from build123d import *

# Parameters (mm, degrees)
SKETCH1_W              = 38.1
SKETCH1_H              = 25.4
BOSS_EXTRUDE1_DEPTH    = 22.225
F_10_CLEARANCE_HOLE1_D = 5.1054
CHAMFER1_SIZE          = 3.175
SKETCH6_W              = 6.35
SKETCH6_H              = 6.35
BOSS_EXTRUDE3_DEPTH    = 6.35
CUT_EXTRUDE1_REACH     = 38.753
SKETCH7_W              = 4.5
SKETCH7_H              = 3.175
CHAMFER4_SIZE          = 1.5875
CHAMFER5_SIZE          = 1.5875
FILLET2_R              = 0.79375


with BuildPart() as part:
    # Sketch1 → Boss-Extrude1 (new body)
    with BuildSketch(Plane(origin=(0, 0, 0), x_dir=(1, 0, 0), z_dir=(0, 1, 0))):
        Rectangle(SKETCH1_W, SKETCH1_H)
    extrude(amount=BOSS_EXTRUDE1_DEPTH)

    # #10 Clearance Hole1 (through all)
    with Locations(Plane(origin=(0, 22.225, 0), x_dir=(1, 0, 0), z_dir=(0, 1, 0))):
        with Locations((-12.7, 0), (12.7, 0)):
            Hole(F_10_CLEARANCE_HOLE1_D / 2)

    # Chamfer1
    chamfer1_edges = [part.edges().sort_by_distance(p)[0] for p in [
        (19.05, 11.1125, 12.7),
        (-19.05, 11.1125, 12.7),
        (-19.05, 11.1125, -12.7),
        (19.05, 11.1125, -12.7),
    ]]
    chamfer(chamfer1_edges, length=CHAMFER1_SIZE)

    # Sketch6 → Boss-Extrude3 (add)
    with BuildSketch(Plane.XY.offset(12.7)):
        with Locations((0, 3.175)):
            Rectangle(SKETCH6_W, SKETCH6_H)
    extrude(amount=BOSS_EXTRUDE3_DEPTH)

    # Sketch7 → Cut-Extrude1 (cut, up to next)
    with BuildSketch(Plane.ZY.offset(3.175), mode=Mode.PRIVATE) as cut_extrude1_sk1:
        with Locations((14.95, 3.175)):
            Rectangle(SKETCH7_W, SKETCH7_H)
    cut_extrude1_tool1 = extrude(cut_extrude1_sk1.sketch, amount=-CUT_EXTRUDE1_REACH, mode=Mode.PRIVATE) & part.part
    add(cut_extrude1_tool1.solids().sort_by_distance((-3.175, 3.175, 14.95))[0], mode=Mode.SUBTRACT)

    # Chamfer4
    chamfer4_edges = [part.edges().sort_by_distance(p)[0] for p in [
        (0, 0, 19.05),
        (0, 6.35, 19.05),
    ]]
    chamfer(chamfer4_edges, length=CHAMFER4_SIZE)

    # Chamfer5
    chamfer5_edges = [part.edges().sort_by_distance(p)[0] for p in [
        (-3.175, 5.55625, 12.7),
        (3.175, 0.79375, 12.7),
        (0, 6.35, 12.7),
        (3.175, 5.55625, 12.7),
        (-3.175, 0.79375, 12.7),
    ]]
    chamfer(chamfer5_edges, length=CHAMFER5_SIZE)

    # Fillet2
    fillet2_edges = [part.edges().sort_by_distance(p)[0] for p in [
        (0, 4.7625, 17.2),
        (0, 1.5875, 17.2),
        (0, 1.5875, 12.7),
        (0, 4.7625, 12.7),
    ]]
    fillet(fillet2_edges, radius=FILLET2_R)


solid = part.part
The model under review builds one solid part; all positions refer to its coordinate system, in mm. A direction names the side the tool comes from. Coordinates: 2 decimals unless noted, no trailing zeros. Write each loop counter-clockwise with the first axis right and the second up, starting at its lowest first coordinate (ties: lowest second). Pieces come first, ordered by that corner, then holes. Notation, with made-up numbers: (0.5, 31) - (53.5, 31) arc R19 ccw to (53.5, 58) - close; hole circle Ø11 at (-21, 18). An arc over 180 degrees is marked (long way). Answer as CSV lines item,"result".
(1) Mouldability with a two-part tool opening along Z and no side actions: class faces 1 (the flat face through (-19.05, 11, 0)), 2 (the flat face through (0, 4.762, 15)), 3 (the flat face through (3.96, 0.91, 13.5)), 4 (the flat face through (-17.44, 10.957, -11.135)) as pulls with the +Z half, pulls with the -Z half, needs draft (parallel to the pull), parting line crosses it, or undercut.
Data:
face 1,"needs draft"
face 2,"undercut"
face 3,"pulls with the +Z half"
face 4,"pulls with the -Z half"
(2) Clearance check with flat-ended pins moving along their axes: pin 1 Ø2.5 at (y, z) = (2.5, 16) entering from -X (3 decimals); pin 2 Ø5 at (y, z) = (4, 16.5) entering from +X; pin 3 Ø1.5 at (x, z) = (-1, 15) entering from +Y; pin 4 Ø3 at (x, z) = (-12.7, 0) entering from -Y. State where each tip first meets the part, or that it passes through.
Data:
pin 1,"stops at x = -3.175"
pin 2,"stops at x = 3.34"
pin 3,"stops at y = 6.39"
pin 4,"passes through"
(3) For line 1 along Z through (x, y) = (12.7, 17.75); line 2 along Z through (x, y) = (-0.5, 14.5); line 3 along Z through (x, y) = (0, 7.5), list the stretches that pass through material, from the lowest coordinate up. Write a range as [from, to].
Data:
line 1,"z = [-12.7, -2.55], [2.55, 12.7]"
line 2,"z = [-12.7, 12.7]"
line 3,"z = [-12.7, 13.14]"
(4) Tool access review of faces 5 (the flat face through (3.175, 3, 18)), 6 (the flat face through (-3.98, 0.91, 13.48)), 7 (the flat face through (0, 6.35, 16)): name each direction out of +Z, -Z, +X, -X, +Y, -Y from which nothing blocks a thin tool from reaching the whole face with its end or side.
Data:
face 5,"+Z, +X, +Y, -Y"
face 6,"+Z, -X, +Y, -Y"
face 7,"+Z, +X, -X, +Y"
(5) We need section B-B (x = -12.7). Give the boundary of the cut face in (y, z) (3 decimals).
Data:
outline,"(0, -12.7) - (22.225, -12.7) - (22.225, -2.553) - (0, -2.553) - close; (0, 2.553) - (22.225, 2.553) - (22.225, 12.7) - (0, 12.7) - close"
(6) We need section C-C (y = 10.25). Give the boundary of the cut face in (x, z) (3 decimals).
Data:
outline,"(-19.05, -9.525) - (-15.875, -12.7) - (15.875, -12.7) - (19.05, -9.525) - (19.05, 9.525) - (15.875, 12.7) - (-15.875, 12.7) - (-19.05, 9.525) - close; hole circle Ø5.105 at (-12.7, 0); hole circle Ø5.105 at (12.7, 0)"
(7) We need section A-A (z = 0). Give the boundary of the cut face in (x, y) (3 decimals), plus the area to 3 significant figures.
Data:
outline,"(-19.05, 0) - (-15.253, 0) - (-15.253, 22.225) - (-19.05, 22.225) - close; (-10.147, 0) - (10.147, 0) - (10.147, 22.225) - (-10.147, 22.225) - close; (15.253, 0) - (19.05, 0) - (19.05, 22.225) - (15.253, 22.225) - close"
area,"620 mm2"
